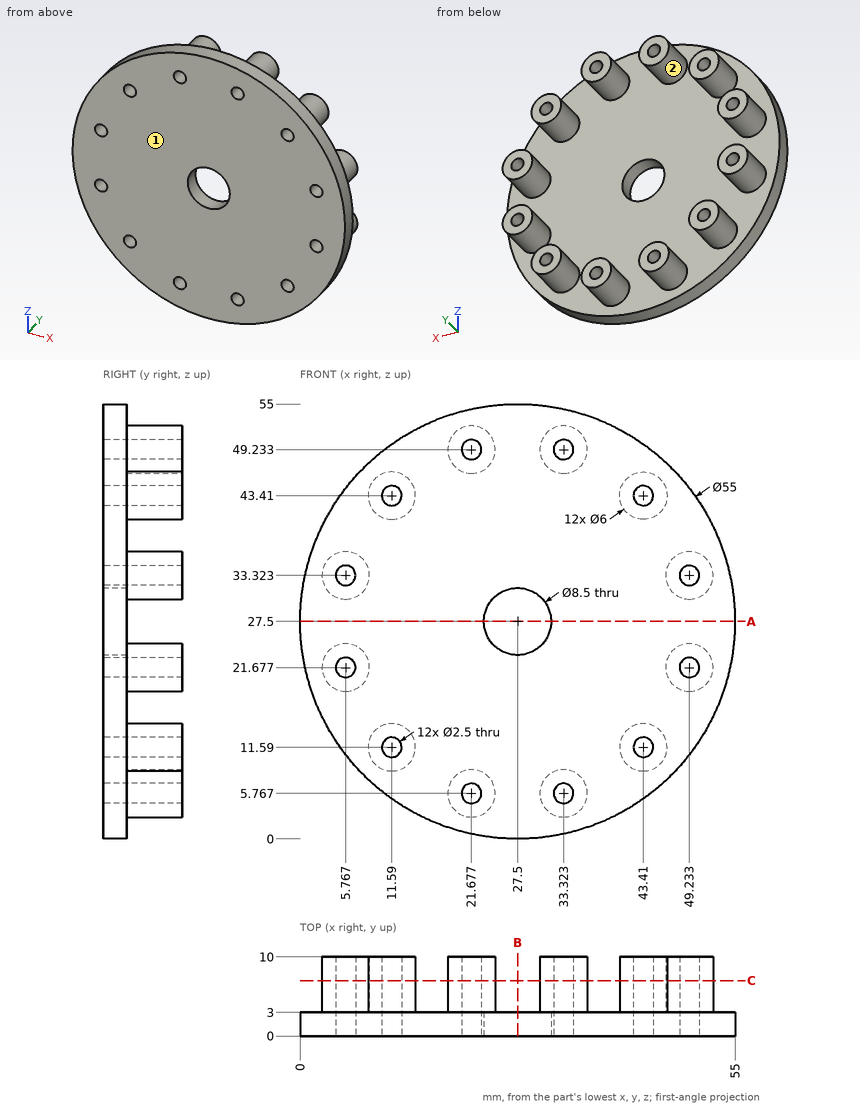
Check sheet for the drawn part. Datum: minimum x, y, z corner. Units: mm. Coordinates: 2 decimals unless noted, no trailing zeros. Order: outer loops, then holes, each group sorted by start corner. A loop starts at its lowest first (then second) coordinate and runs counter-clockwise, first axis right, second up. Notation, with made-up numbers: M 0,47 L 51,47 A16 ccw 51,62 Z; hole C 10,-7.75 d1. An arc over 180 degrees is marked long. One line per item, written item: value. Start each with the question number.
Item 1: Scan lines: probe 1 along X at (y, z) = (2.25, 43) (1 decimal); probe 2 along Z at (x, y) = (6.5, 3.5) (1 decimal); probe 3 along X at (y, z) = (4, 21) (1 decimal). Record each from-to range of solid material in increasing order.
Item 2: Sectioned sample at C-C (y = 7). Count the separate pieces of the cut face and the enclosed holes in it.
Item 3: Mould release check, pull along X, two halves, no side actions. Record for the marked faces 1 and 2: released by +X, released by -X, zero draft, split by the parting line, or undercut.
Item 4: Gauge pin test, flat ends, axial feed: pin 1 (4 mm diameter, centred on x = 25, y = 6, fed in from +Z) (1 decimal); pin 2 (1.5 mm diameter, centred on y = 2.5, z = 41, fed in from -X) (1 decimal). Record the tip position at first contact, or that the pin passes through.
Item 5: Sectioned sample at B-B (x = 27.5). Enter the section's corners in (y, z).
Item 6: Sectioned sample at A-A (z = 27.5). Enter the section's corners in (x, y).
Conclusion:
1. probe 1: x = 4.8 to 10.4, 12.8 to 42.2, 44.6 to 50.2
1. probe 2: z = 18.8 to 20.7, 22.7 to 24.6, 30.4 to 32.3, 34.3 to 36.2
1. probe 3: x = 2.8 to 4.7, 6.8 to 8.7, 46.3 to 48.2, 50.3 to 52.2
2. separate pieces: 12
2. enclosed holes: 12
3. face 1: zero draft
3. face 2: undercut
4. pin 1: stops at z = 51.9
4. pin 2: stops at x = 3.1
5. outline: M 0,0 L 3,0 L 3,23.25 L 0,23.25 Z; M 0,31.75 L 3,31.75 L 3,55 L 0,55 Z
6. outline: M 0,0 L 23.25,0 L 23.25,3 L 0,3 Z; M 31.75,0 L 55,0 L 55,3 L 31.75,3 Z
